from build123d import *

# Parameters (mm, degrees)
SKETCH1_R           = 2.4892
BOSS_EXTRUDE1_DEPTH = 3.175
LPATTERN1_START     = -3.175
LPATTERN1_OUTLINE_R = 2.4892
LPATTERN1_DEPTH     = 6.35
SKETCH2_R           = 2.4892
CUT_EXTRUDE1_DEPTH  = 123.679962198
FILLET1_R           = 6.35


# Read off the part's stored shape, not the designer's step: LPattern1
with BuildPart() as part:
    # Sketch1 → Boss-Extrude1 (new, symmetric)
    with BuildSketch(Plane.XY):
        Polygon((0, 104.775), (25.4, 104.775), (63.5, 50.8), (63.5, 0), (0, 0), (-38.1, 0), (-38.1, 50.8), align=None)
        with Locations((12.7, 85.725)):
            Circle(SKETCH1_R, mode=Mode.SUBTRACT)
        with Locations((12.7, 73.025)):
            Circle(SKETCH1_R, mode=Mode.SUBTRACT)
        with Locations((12.7, 12.7)):
            Circle(SKETCH1_R, mode=Mode.SUBTRACT)
    extrude(amount=BOSS_EXTRUDE1_DEPTH, both=True)

    # LPattern1 outline → LPattern1 (cut)
    with BuildSketch(Plane.XY.offset(LPATTERN1_START)):
        with Locations((50.8, 38.1)):
            Circle(LPATTERN1_OUTLINE_R)
        with Locations((38.1, 38.1)):
            Circle(LPATTERN1_OUTLINE_R)
        with Locations((25.4, 38.1)):
            Circle(LPATTERN1_OUTLINE_R)
        with Locations((12.7, 38.1)):
            Circle(LPATTERN1_OUTLINE_R)
        with Locations((50.8, 25.4)):
            Circle(LPATTERN1_OUTLINE_R)
        with Locations((38.1, 25.4)):
            Circle(LPATTERN1_OUTLINE_R)
        with Locations((25.4, 25.4)):
            Circle(LPATTERN1_OUTLINE_R)
        with Locations((12.7, 25.4)):
            Circle(LPATTERN1_OUTLINE_R)
        with Locations((50.8, 12.7)):
            Circle(LPATTERN1_OUTLINE_R)
        with Locations((38.1, 12.7)):
            Circle(LPATTERN1_OUTLINE_R)
        with Locations((25.4, 12.7)):
            Circle(LPATTERN1_OUTLINE_R)
    extrude(amount=LPATTERN1_DEPTH, mode=Mode.SUBTRACT)

    # Sketch2 → Cut-Extrude1 (cut, through all)
    with BuildSketch(Plane.XY.offset(3.175)):
        with Locations((12.7, 38.1)):
            Circle(SKETCH2_R)
        with Locations((12.7, 25.4)):
            Circle(SKETCH2_R)
        with Locations((12.7, 12.7)):
            Circle(SKETCH2_R)
        with Locations((0, 12.7)):
            Circle(SKETCH2_R)
        with Locations((0, 25.4)):
            Circle(SKETCH2_R)
        with Locations((0, 38.1)):
            Circle(SKETCH2_R)
        with Locations((-12.7, 12.7)):
            Circle(SKETCH2_R)
        with Locations((-12.7, 25.4)):
            Circle(SKETCH2_R)
        with Locations((-12.7, 38.1)):
            Circle(SKETCH2_R)
        with Locations((-25.4, 12.7)):
            Circle(SKETCH2_R)
        with Locations((-25.4, 25.4)):
            Circle(SKETCH2_R)
        with Locations((-25.4, 38.1)):
            Circle(SKETCH2_R)
        Polygon((25.4, 50.8), (25.4, 93.763754959), (55.727356441, 50.8), align=None)
        Polygon((0, 50.8), (-30.327356441, 50.8), (0, 93.763754959), align=None)
    extrude(amount=-CUT_EXTRUDE1_DEPTH, mode=Mode.SUBTRACT)

    # Fillet1
    fillet1_edges = [part.edges().sort_by_distance(p)[0] for p in [
        (-38.1, 0, 0),
        (-38.1, 50.8, 0),
        (0, 104.775, 0),
        (25.4, 104.775, 0),
        (63.5, 50.8, 0),
        (63.5, 0, 0),
        (55.727356441, 50.8, 0),
        (25.4, 50.8, 0),
        (25.4, 93.763754959, 0),
        (0, 93.763754959, 0),
        (0, 50.8, 0),
        (-30.327356441, 50.8, 0),
    ]]
    fillet(fillet1_edges, radius=FILLET1_R)


solid = part.part
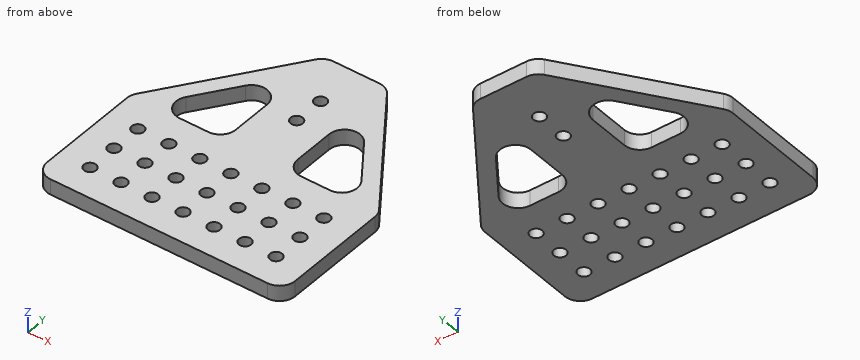
Design review of the part built by this model. Coordinates are the model's own, in mm. Give positions to 0.01 mm unless a question says otherwise; leave off trailing zeros. Loops run counter-clockwise (first coordinate to the right, second up) from the corner with the lowest first, then second, coordinate; pieces in that order, holes last. Notation, with made-up numbers: (-17.5, 75) - (8.5, 75) arc R18 ccw to (8.5, 80) - close; hole circle Ø2 at (87, -27). An arc over 180 degrees is marked (long way). Use CSV: the item, a comma, the result in double quotes. Start each with the question number.
1. Insertion check: P1, Ø1.9, axis at y = 64, z = 1, coming from the +X side; P2, Ø1.9, axis at x = -12, z = 0, coming from the +Y side. Each pin has a flat end and moves straight along its axis. Give the tip position at first contact, or say it passes through.
2. Wall thickness on L1, parallel to Y at x = 12.7, z = 0 (3 decimals); L2, parallel to Y at x = 50.8, z = -2; L3, parallel to Y at x = 37, z = -0.5: over which ranges is each line inside the solid? List them lowest first.
3. Add section B-B (x = 47). State the section outline as (y, z) points (3 decimals).
4. Add section A-A (y = 25.4). Count the separate pieces of the cut face and the enclosed holes in it, plus the area to 3 significant figures.
Results found:
1,P1,"stops at x = 54.85"
1,P2,"stops at y = 89.12"
2,L1,"y = 0 to 10.211, 15.189 to 22.911, 27.889 to 35.611, 40.589 to 70.536, 75.514 to 83.236, 88.214 to 104.775"
2,L2,"y = 0 to 10.21, 15.19 to 22.91, 27.89 to 35.61, 40.59 to 68.79"
2,L3,"y = 0 to 10.47, 14.93 to 23.17, 27.63 to 35.87, 40.33 to 50.8, 77.33 to 88.34"
3,outline,"(0, -3.175) - (51.87, -3.175) - (51.87, 3.175) - (0, 3.175) - close; (63.164, -3.175) - (74.175, -3.175) - (74.175, 3.175) - (63.164, 3.175) - close"
4,separate pieces,"8"
4,enclosed holes,"0"
4,area,"424 mm²"
